Answer from the drawing. Dimensions are ordinates in mm from the lowest x, y and z of the part. A direction names the side the tool comes from. Round coordinates to 2 decimals unless told otherwise and drop trailing zeros. Loops run counter-clockwise (first coordinate to the right, second up) from the corner with the lowest first, then second, coordinate; pieces in that order, holes last. Notation, with made-up numbers: (84.25, -18) - (142.25, -18) arc R29 cw to (142.25, 16) - close; hole circle Ø3 at (-30.5, 49.5). An arc over 180 degrees is marked (long way). Return JSON: item names as keys, results as strings.
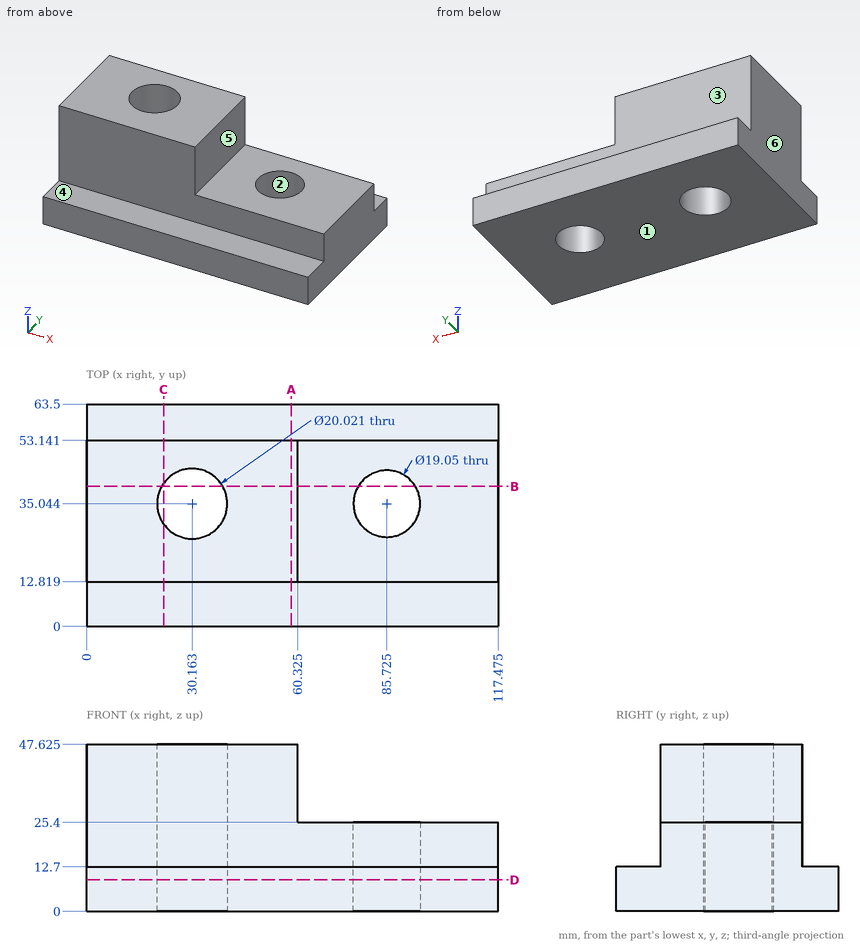
1) Section B-B (y = 40) is taken. Give the vertices of the cut face in (x, z) (1 decimal).
Verdict:
{"outline": "(0, 0) - (21.5, 0) - (21.5, 47.6) - (0, 47.6) - close; (38.9, 0) - (77.6, 0) - (77.6, 25.4) - (60.3, 25.4) - (60.3, 47.6) - (38.9, 47.6) - close; (93.9, 0) - (117.5, 0) - (117.5, 25.4) - (93.9, 25.4) - close"}
2) Find the intervals of material crossed by L1, parallel to Y at x = 86, z = 12 (1 decimal); L2, parallel to X at y = 18.5, z = 44 (1 decimal); L3, parallel to Z at x = 37.5, y = 54, in increasing order.
Verdict:
{"L1": "y = 0 to 25.5, 44.6 to 63.5", "L2": "x = 0 to 60.3", "L3": "z = 0 to 12.7"}
3) Section D-D (z = 9) is taken. Count the separate pieces of the cut face and the enclosed holes in it, and give its area (3 significant figures).
Verdict:
{"separate pieces": "1", "enclosed holes": "2", "area": "6,860 mm2"}
4) Section A-A (x = 58.5) is taken. Give the vertices of the cut face in (y, z) (1 decimal).
Verdict:
{"outline": "(0, 0) - (63.5, 0) - (63.5, 12.7) - (53.1, 12.7) - (53.1, 47.6) - (12.8, 47.6) - (12.8, 12.7) - (0, 12.7) - close"}
5) Section C-C (x = 22) is taken. Give the vertices of the cut face in (y, z) (1 decimal), and give its area (3 significant figures).
Verdict:
{"outline": "(0, 0) - (29.2, 0) - (29.2, 47.6) - (12.8, 47.6) - (12.8, 12.7) - (0, 12.7) - close; (40.8, 0) - (63.5, 0) - (63.5, 12.7) - (53.1, 12.7) - (53.1, 47.6) - (40.8, 47.6) - close", "area": "1,660 mm2"}
6) Determine the mould class of the marked faces 1, 2 and 3 for opening direction Y: pulls with the +Y half, pulls with the -Y half, needs draft (parallel to the pull), parting line crosses it, or undercut.
Verdict:
{"face 1": "needs draft", "face 2": "undercut", "face 3": "pulls with the +Y half"}
7) A tool of negligible diameter and unlimited length cuts with its end or side. For the marked faces 4, 5 and 6, from which of +Z, -Z, +X, -X, +Y, -Y can it reach the whole face along a straight path? Write none if from no direction.
Verdict:
{"face 4": "+Z, +X, -X, -Y", "face 5": "+Z, +X, +Y, -Y", "face 6": "+Z, -Z, -X, +Y, -Y"}
8) Flat-ended cylindrical pins translate along their axes: pin 1 (12 mm diameter, centred on x = 93, y = 25.5, fed in from +Z); pin 2 (3 mm diameter, centred on x = 17, y = 9.5, fed in from +Z); pin 3 (6 mm diameter, centred on x = 29, z = 24, fed in from -Y). Find the tip coordinate at first contact, or state that the pin passes through.
Verdict:
{"pin 1": "stops at z = 25.4", "pin 2": "stops at z = 12.7", "pin 3": "stops at y = 12.82"}
